Build history of the part. All positions in model axes, mm. A direction names the side the tool comes from. Give positions to 0.01 mm unless a question says otherwise; leave off trailing zeros. Loops run counter-clockwise (first coordinate to the right, second up) from the corner with the lowest first, then second, coordinate; pieces in that order, holes last. Notation, with made-up numbers: M -32,20.25 L -13,20.25 A24 ccw -13,43.25 Z; hole C 40.25,87.5 d5. An arc over 180 degrees is marked long. Answer as a JSON object with one key per item and string values. Group by question number.
1. Slice it at B-B (y = 6.25). List the corners of the cut face in (x, z) (3 decimals).
2. Slice it at A-A (z = -9). List the corners of the cut face in (x, y), then the cut area to 3 significant figures.
3. 3-axis set-ups, long thin cutter, end or side, ignore diameter. For faces 4 (the face through (-41.274, 3.757, 0.222)), 5 (the face through (0.327, 2.504, 70.482)): which of +Z, -Z, +X, -X, +Y, -Y reach the whole face in a straight line?
4. Drill centre lines: line 1 along X through (y, z) = (1.5, 0) (3 decimals); line 2 along Y through (x, z) = (-3, 59); line 3 along Z through (x, y) = (-1, 2.75). Where is each one in solid material? Low to high. Write a range as [from, to].
5. Drop flat-ended pins along their axis: pin 1 Ø1.5 at (x, y) = (-20.5, 1) entering from -Z; pin 2 Ø3 at (y, z) = (3.5, 35) entering from -X; pin 3 Ø1 at (y, z) = (4.5, -14) entering from +X. Give the stop position or say it passes through.
6. Mould opens along Z. For faces 1 (the face through (1, 7.62, 1)), 2 (the face through (-27.2, 2.5, 36.05)), 3 (the face through (-29.557, 3.757, -37.001)) say: released by +Z, released by -Z, zero draft, split by the parting line, or undercut.
Autodesk Inventor part; units mm, degrees
ref_plane "YZ Plane" through (0, 0, 0) normal (1, 0, 0) x (0, 1, 0)
ref_plane "XZ Plane" through (0, 0, 0) normal (0, 1, 0) x (-1, 0, 0)
ref_plane "XY Plane" through (0, 0, 0) normal (0, 0, 1) x (1, 0, 0)
sketch "Sketch1" plane through (0, 0, 0) normal (0, 1, 0) x (-1, 0, 0)
  circle A0 centre (0, 0) radius 41.275
  circle A1 centre (0, 50.8) radius 22.225
  circle A2 centre (0, -50.8) radius 22.225
  line L0 (38.2629, 15.4781) -> (20.6031, 59.1344)
  line L1 (-38.2629, 15.4781) -> (-20.6031, 59.1344)
  line L2 (-38.2629, -15.4781) -> (-20.6031, -59.1344)
  line L3 (38.2629, -15.4781) -> (20.6031, -59.1344)
  dimension "d0" = 82.55
  dimension "d1" = 44.45
  dimension "d2" = 44.45
  dimension "d3" = 50.8
  dimension "d4" = 50.8
extrude "Extrusion1" add sketch "Sketch1" along normal blind 7.62
shell "Shell2" thickness 2.54 removed faces 1 at (-6.8677, 0, -30.0302)
properties part number "Diamond-Box-Lid"
Established:
{
 "1": {"outline": "M -38.263,-15.478 L -20.603,-59.134 A22.225 ccw 20.603,-59.134 L 38.263,-15.478 A41.275 ccw 38.263,15.478 L 20.603,59.134 A22.225 ccw -20.603,59.134 L -38.263,15.478 A41.275 ccw Z"},
 "2": {"outline": "M -40.28,0 L -37.67,0 L -37.67,5.08 L 37.67,5.08 L 37.67,0 L 40.28,0 L 40.28,7.62 L -40.28,7.62 Z", "area": "231 mm^2"},
 "3": {"face 4": "-X, +Y, -Y", "face 5": "-Y"},
 "4": {"line 1": "x = [-41.275, -38.735], [38.735, 41.275]", "line 2": "y = [5.08, 7.62]", "line 3": "z = [-73, -70.46], [70.46, 73]"},
 "5": {"pin 1": "stops at z = -60.99", "pin 2": "stops at x = -30.97", "pin 3": "stops at x = 39"},
 "6": {"face 1": "zero draft", "face 2": "undercut", "face 3": "released by -Z"}
}
